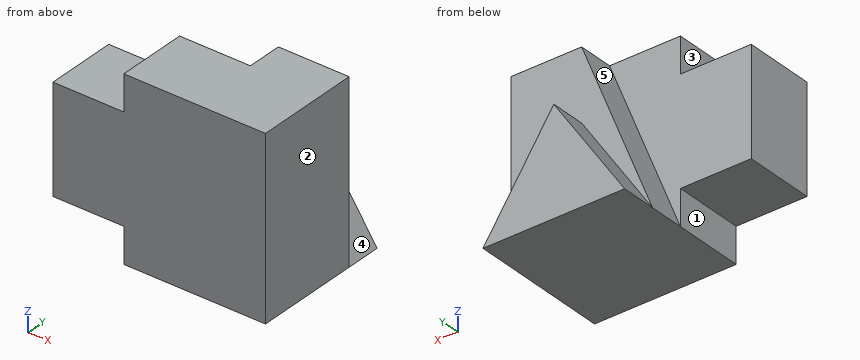
```python
from build123d import *

# Parameters (mm, degrees)
BOSS_EXTRUDE1_DEPTH = 25
SKETCH2_W           = 15
SKETCH2_H           = 10
BOSS_EXTRUDE2_DEPTH = 10
SKETCH3_W           = 25
SKETCH3_H           = 10
BOSS_EXTRUDE3_DEPTH = 10
CUT_EXTRUDE1_DEPTH  = 5
CUT_EXTRUDE2_DEPTH  = 5


with BuildPart() as part:
    # Sketch1 → Boss-Extrude1 (new body)
    with BuildSketch(Plane.XY):
        Polygon((0, 0), (20, 0), (20, 20), (10, 20), (10, 10), (0, 10), align=None)
    extrude(amount=BOSS_EXTRUDE1_DEPTH)

    # Sketch2 → Boss-Extrude2 (add)
    with BuildSketch(Plane.ZY):
        with Locations((12.5, 5)):
            Rectangle(SKETCH2_W, SKETCH2_H)
    extrude(amount=BOSS_EXTRUDE2_DEPTH)

    # Sketch3 → Boss-Extrude3 (add)
    with BuildSketch(Plane.ZY.offset(-10)):
        with Locations((12.5, 15)):
            Rectangle(SKETCH3_W, SKETCH3_H)
    extrude(amount=BOSS_EXTRUDE3_DEPTH)

    # Sketch5 → Cut-Extrude1 (cut)
    with BuildSketch(Plane(origin=(0, 20, 0), x_dir=(1, 0, 0), z_dir=(0, 1, 0))):
        Polygon((0, 0), (0, -25), (20, -25), (20, 0), (10, -15), align=None)
    extrude(amount=-CUT_EXTRUDE1_DEPTH, mode=Mode.SUBTRACT)

    # Sketch6 → Cut-Extrude2 (cut)
    with BuildSketch(Plane(origin=(0, 15, 0), x_dir=(1, 0, 0), z_dir=(0, 1, 0))):
        Polygon((0, -25), (10, -25), (0, 0), align=None)
    extrude(amount=-CUT_EXTRUDE2_DEPTH, mode=Mode.SUBTRACT)


solid = part.part
```
Work out the finished part from the listing and answer in its coordinate system (mm). Face numbers are marked on the shaded views. A direction names the side the tool comes from. Round coordinates to 2 decimals unless told otherwise and drop trailing zeros. Write each loop counter-clockwise with the first axis right and the second up, starting at its lowest first coordinate (ties: lowest second). Pieces come first, ordered by that corner, then holes. Notation, with made-up numbers: (-2.5, 38.5) -> (14.5, 38.5) arc R9 ccw to (14.5, 47.5) -> close; hole circle Ø4 at (-8, 30). An arc over 180 degrees is marked (long way). Write each question's results on one line, items separated by ' | '.
Q1. Section A-A, the plane z = 12 is taken. Write down the section's boundary in (x, y).
Data:
outline: (-10, 0) -> (20, 0) -> (20, 15) -> (12, 15) -> (12, 20) -> (8, 20) -> (8, 15) -> (4.8, 15) -> (4.8, 10) -> (-10, 10) -> close
Q2. Which of the six approach directions +Z, -Z, +X, -X, +Y, -Y give full straight-line access (tool end or side, diameter ignored) to the marked faces 1, 2, 3, 4 and 5?
Data:
face 1: -Z, -X, +Y, -Y | face 2: +Z, -Z, +X, +Y, -Y | face 3: +Z, -X, +Y, -Y | face 4: +Z, +X, +Y | face 5: +Z, -X, +Y
Q3. Section B-B, the plane y = 6.25 is taken. Write down the section's boundary in (x, z).
Data:
outline: (-10, 5) -> (0, 5) -> (0, 0) -> (20, 0) -> (20, 25) -> (0, 25) -> (0, 20) -> (-10, 20) -> close
Q4. Straight lines are drawn through the part: line 1 along Y through (x, z) = (17.5, 21.25); line 2 along Z through (x, y) = (-2, 9.25); line 3 along Y through (x, z) = (1.75, 23). For each, find the intervals that lie inside material, in ascending order. Write a range as [from, to].
Data:
line 1: [0, 15] | line 2: [5, 20] | line 3: [0, 10]
Q5. Section C-C, the plane x = 6.5 is taken. Write down the section's boundary in (y, z).
Data:
outline: (0, 0) -> (20, 0) -> (20, 9.75) -> (15, 9.75) -> (15, 16.25) -> (10, 16.25) -> (10, 25) -> (0, 25) -> close
Q6. Section D-D, the plane z = 6 is taken. Write down the section's boundary in (x, y), then the cut area to 3 significant figures.
Data:
outline: (-10, 0) -> (20, 0) -> (20, 15) -> (16, 15) -> (16, 20) -> (4, 20) -> (4, 15) -> (2.4, 15) -> (2.4, 10) -> (-10, 10) -> close | area: 448 mm^2
Q7. Flat-ended cylindrical pins translate along their axes: P1, Ø4, axis at y = 5, z = 23.5, coming from the -X side; P2, Ø5, axis at x = -6, y = 5.5, coming from the +Z side; P3, Ø5, axis at x = -7, y = 3, coming from the -Z side. Find the tip coordinate at first contact, or state that the pin passes through.
Data:
P1: x = 0 | P2: z = 20 | P3: z = 5
